The model under review builds one solid part; all positions refer to its coordinate system, in mm. Give positions to 0.01 mm unless a question says otherwise; leave off trailing zeros. Order: outer loops, then holes, each group sorted by start corner. A loop starts at its lowest first (then second) coordinate and runs counter-clockwise, first axis right, second up. Notation, with made-up numbers: (0, 83) - (17, 83) arc R19 cw to (17, 111) - close; hole circle Ø4 at (-30, 68). An arc over 180 degrees is marked (long way). Use a Markdown table: item, result. Add a question column.
```python
from build123d import *

# Parameters (mm, degrees)
F0_W     = 200
F0_H     = 200
F1_DEPTH = 25
F3_DEPTH = 25
F4_R     = 25
F5_REACH = 228.5588830885
F7_REACH = 193.2035440291
F8_R     = 21
F9_DEPTH = 101.0840931723


with BuildPart() as f1:
    # F0 (on Front) → F1 (new body)
    with BuildSketch(Plane.XZ):
        Rectangle(F0_W, F0_H)
    extrude(amount=F1_DEPTH)

    # F2 (on Right) → F3 (join)
    with BuildSketch(Plane.YZ):
        Polygon((-74.9957839266, 48.9940974972), (-25, 0), (-25, 70.0059030005), (-40, 84.7053717305), align=None)
    extrude(amount=F3_DEPTH)

    f5_end = Plane(origin=(-0.5719458586, -25, -1.601583452), x_dir=(0, 0, -1), z_dir=(0, -1, 0))
    # F4 (on face) → F5 (join, up to a plane its end follows)
    with BuildSketch(Plane(origin=(0, -62.7487350002, 61.4915378653), x_dir=(1, 0, 0), z_dir=(0, -0.7142254847, 0.6999156785))):
        with Locations((0, 7.5021080367)):
            Circle(F4_R)
    f5_long = extrude(amount=-F5_REACH, mode=Mode.PRIVATE)
    add(split(f5_long, bisect_by=f5_end, keep=Keep.TOP, mode=Mode.PRIVATE))

    f7_end = Plane(origin=(-0.1977552343, -25, -2.9660534924), x_dir=(0, 0, -1), z_dir=(0, -1, 0))
    # F6 (on face) → F7 (cut, up to a plane its end follows)
    with BuildSketch(Plane(origin=(0, -62.7487350002, 61.4915378653), x_dir=(1, 0, 0), z_dir=(0, -0.7142254847, 0.6999156785))):
        with BuildLine():
            ThreePointArc((0, 32.5021080367), (17.6776695297, 25.1797775664), (25, 7.5021080367))
            Line((25, 7.5021080367), (25, 32.5021080367))
            Line((25, 32.5021080367), (0, 32.5021080367))
        make_face()
        with BuildLine():
            ThreePointArc((25, 7.5021080367), (17.6776695297, -10.175561493), (0, -17.4978919633))
            Line((0, -17.4978919633), (25, -17.4978919633))
            Line((25, -17.4978919633), (25, 7.5021080367))
        make_face()
    f7_long = extrude(amount=-F7_REACH, mode=Mode.PRIVATE)
    add(split(f7_long, bisect_by=f7_end, keep=Keep.TOP, mode=Mode.PRIVATE), mode=Mode.SUBTRACT)

    # F8 (on face) → F9 (cut, through all)
    with BuildSketch(Plane(origin=(0, -62.7487350002, 61.4915378653), x_dir=(1, 0, 0), z_dir=(0, -0.7142254847, 0.6999156785))):
        with Locations((0, 7.5021080367)):
            Circle(F8_R)
    extrude(amount=-F9_DEPTH, mode=Mode.SUBTRACT)


solid = f1.part
```
Q1. We need section C-C (x = 53). Write out the cut boundary in (y, z).
Q2. Clearance check with flat-ended pins moving along their axes: P1, Ø1, axis at y = -40.5, z = 57, coming from the +X side; P2, Ø12, axis at x = 25, y = -63.5, coming from the +Z side; P3, Ø3, axis at x = 9, y = -62.5, coming from the +Z side. State where each tip first meets the part, or that it passes through.
Q3. Draft analysis for pull direction X (two halves, no side actions). For faces 1 (the flat face through (-1, -12, 100)), 2 (the cylindrical face through (-4.552, -44.163, 25.079)), 3 (the flat face through (-100, -12, -1)), state which applies: pulls with the +X half, pulls with the -X half, needs draft (parallel to the pull), parting line crosses it, or undercut.
Q4. We need section B-B (z = -43). Write out the cut boundary in (x, y), plus the area to 3 significant figures.
Q5. We need section A-A (x = 6). Write out the cut boundary in (y, z), plus the area to 3 significant figures.
Q6. Wall thickness on probe 1 along Y at (x, z) = (-46, -23); probe 2 along X at (y, z) = (-9, 23); probe 3 along Z at (x, y) = (-8.5, -42): over which ranges is each line inside the solid? List them lowest first.
Here are the results:
| question | item | result |
|---|---|---|
| 1 | outline | (-25, -100) - (0, -100) - (0, 100) - (-25, 100) - close |
| 2 | P1 | x = 24.62 |
| 2 | P2 | z = 66.85 |
| 2 | P3 | z = 47 |
| 3 | face 1 | needs draft |
| 3 | face 2 | undercut |
| 3 | face 3 | pulls with the -X half |
| 4 | outline | (-100, -25) - (100, -25) - (100, 0) - (-100, 0) - close |
| 4 | area | 5,000 mm2 |
| 5 | outline | (-74.48, 49.52) - (-25, 1.02) - (-25, -100) - (0, -100) - (0, -17.67) - (-71.58, 52.48) - close; (-43.41, 81.22) - (0, 38.68) - (0, 100) - (-25, 100) - (-25, 68.98) - (-40.51, 84.18) - close |
| 5 | area | 3,970 mm2 |
| 6 | probe 1 | -25 to 0 |
| 6 | probe 2 | -100 to -20.84, 20.84 to 100 |
| 6 | probe 3 | 18.74 to 24.78, 78.55 to 82.66 |
